Source: three-view drawing plus pictorial views. Frame: mm from the lowest corner of the part. Give positions to 0.01 mm unless a question says otherwise; leave off trailing zeros. Loops run counter-clockwise (first coordinate to the right, second up) from the corner with the lowest first, then second, coordinate; pieces in that order, holes last. Notation, with made-up numbers: (46, -11.75) - (91, -11.75) arc R14 cw to (91, 9.25) - close; hole circle Ø4 at (73, -35.5). An arc over 180 degrees is marked (long way). Answer in a Markdown table with one row per item.
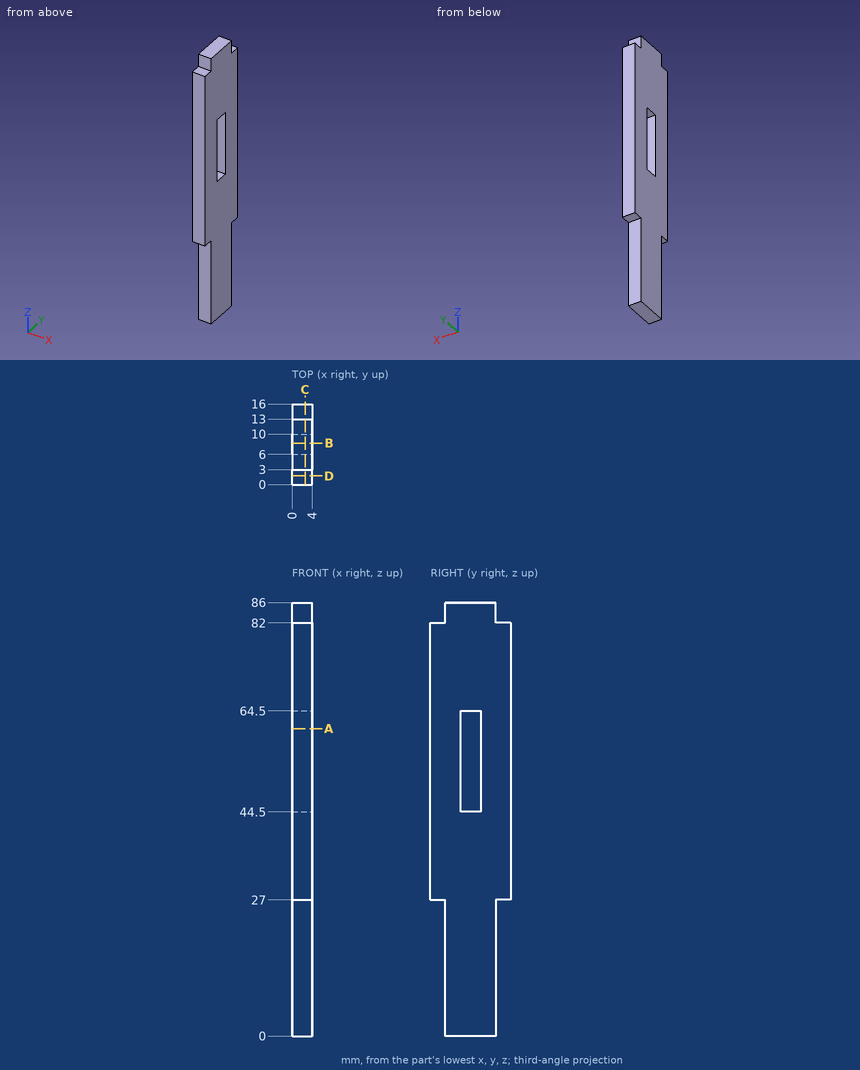
Q1. Cut plane A-A (z = 61). Output: boundary loops of the cut face in (x, y), and give its area (3 significant figures).
Check values:
| item | result |
|---|---|
| outline | (0, 0) - (4, 0) - (4, 6) - (0, 6) - close; (0, 10) - (4, 10) - (4, 16) - (0, 16) - close |
| area | 48.0 mm² |
Q2. Cut plane B-B (y = 8.25). Output: boundary loops of the cut face in (x, z), and give its area (3 significant figures).
Check values:
| item | result |
|---|---|
| outline | (0, 0) - (4, 0) - (4, 44.5) - (0, 44.5) - close; (0, 64.5) - (4, 64.5) - (4, 86) - (0, 86) - close |
| area | 264 mm² |
Q3. Cut plane D-D (y = 1.75). Output: boundary loops of the cut face in (x, z).
Check values:
| item | result |
|---|---|
| outline | (0, 27) - (4, 27) - (4, 82) - (0, 82) - close |
Q4. Material intervals for line 1 along Z through (x, y) = (2.2, 8); line 2 along Y through (x, z) = (2.45, 4); line 3 along Y through (x, z) = (1.25, 50), sorted ascending.
Check values:
| item | result |
|---|---|
| line 1 | 0 to 44.5, 64.5 to 86 |
| line 2 | 3 to 13 |
| line 3 | 0 to 6, 10 to 16 |
Q5. Cut plane C-C (x = 2.6). Output: boundary loops of the cut face in (y, z), and give its area (3 significant figures).
Check values:
| item | result |
|---|---|
| outline | (0, 27) - (3, 27) - (3, 0) - (13, 0) - (13, 27) - (16, 27) - (16, 82) - (13, 82) - (13, 86) - (3, 86) - (3, 82) - (0, 82) - close; hole (6, 44.5) - (10, 44.5) - (10, 64.5) - (6, 64.5) - close |
| area | 1,110 mm² |
Q6. First-contact query: pin 1 (1.2 mm diameter, centred on x = 2, z = 16.5, fed in from -Y); pin 2 (0.9 mm diameter, centred on x = 2, y = 14.5, fed in from +Z). Flat tips, straight axial feed; report the tip coordinate or a pass-through.
Check values:
| item | result |
|---|---|
| pin 1 | y = 3 |
| pin 2 | z = 82 |
